Answer from the drawing. Dimensions are ordinates in mm from the lowest x, y and z of the part. Give positions to 0.01 mm unless a question says otherwise; leave off trailing zeros. Order: outer loops, then holes, each group sorted by start corner. A loop starts at its lowest first (then second) coordinate and runs counter-clockwise, first axis right, second up. Notation, with made-up numbers: (25.25, 28) -> (83.25, 28) arc R19 ccw to (83.25, 57) -> close; hole circle Ø7 at (-10.75, 26). An arc over 180 degrees is marked (long way). One line per question, with ' | ' between items. Start each with the question number.
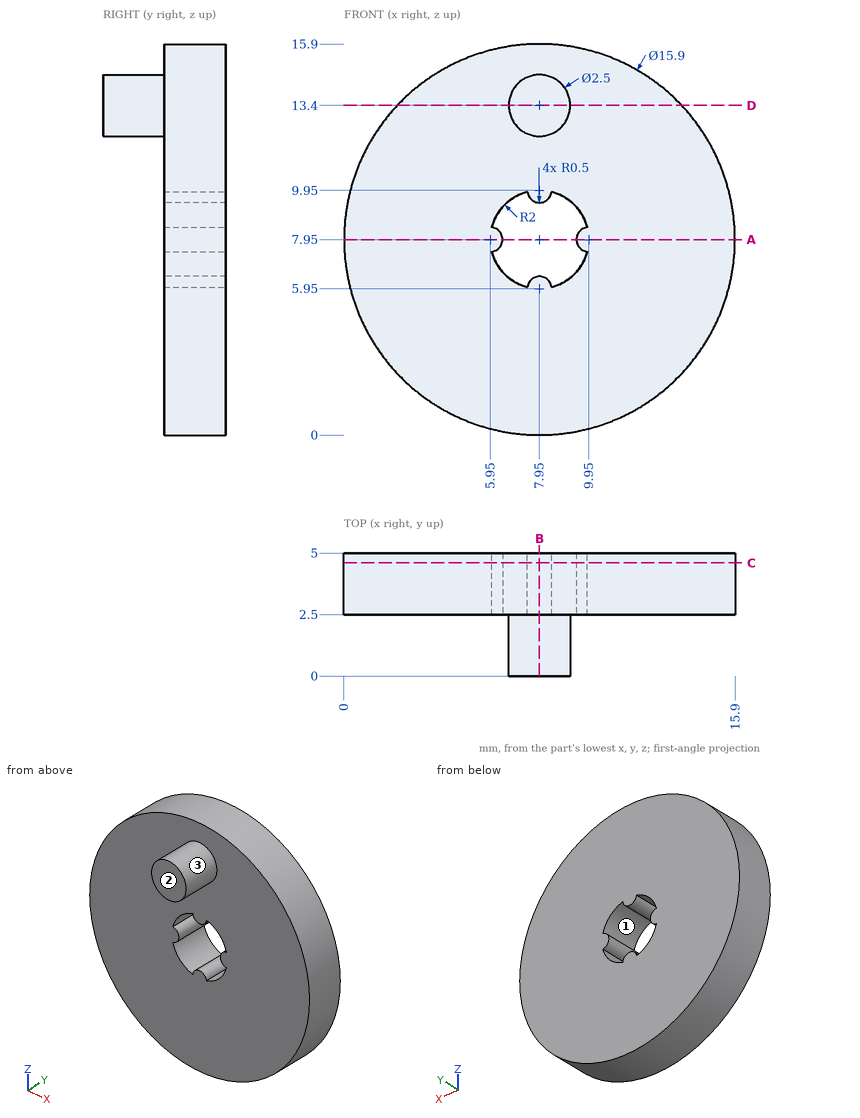
(1) The part is cut by section B-B on x = 7.95. Determine the outline of the cut face in (y, z), plus the area to 3 significant figures.
(2) The part is cut by section A-A on z = 7.95. Determine the outline of the cut face in (x, y).
(3) Given P1, Ø1.5, axis at y = 2, z = 10.5, coming from the -X side; P2, Ø1, axis at x = 10, z = 11, coming from the -Y side, each flat-ended and moving along its own axis, determine where each tip first touches the part or whether it passes through.
(4) The part is cut by section C-C on y = 4.6. Determine the outline of the cut face in (x, z).
(5) The part is cut by section D-D on z = 13.4. Determine the outline of the cut face in (x, y), plus the area to 3 significant figures.
(6) Consider line 1 (Y direction, x = 11.75, z = 3.75); line 2 (Z direction, x = 6.5, y = 4.05); line 3 (X direction, y = 3.25, z = 7). Determine where each line is inside the solid, lowest interval first.
(7) Determine the mould class of the marked faces 1, 2 and 3 for opening direction Z: pulls with the +Z half, pulls with the -Z half, needs draft (parallel to the pull), parting line crosses it, or undercut.
Result sheet:
1) outline: (0, 12.15) -> (2.5, 12.15) -> (2.5, 9.45) -> (5, 9.45) -> (5, 15.9) -> (2.5, 15.9) -> (2.5, 14.65) -> (0, 14.65) -> close; (2.5, 0) -> (5, 0) -> (5, 6.45) -> (2.5, 6.45) -> close | area: 38.5 mm^2
2) outline: (0, 2.5) -> (6.45, 2.5) -> (6.45, 5) -> (0, 5) -> close; (9.45, 2.5) -> (15.9, 2.5) -> (15.9, 5) -> (9.45, 5) -> close
3) P1: stops at x = 0.25 | P2: stops at y = 2.5
4) outline: circle Ø15.9 at (7.95, 7.95); hole (6.01, 7.45) arc R2 ccw to (7.45, 6.01) arc R0.5 cw to (8.45, 6.01) arc R2 ccw to (9.89, 7.45) arc R0.5 cw to (9.89, 8.45) arc R2 ccw to (8.45, 9.89) arc R0.5 cw to (7.45, 9.89) arc R2 ccw to (6.01, 8.45) arc R0.5 cw to start
5) outline: (2.16, 2.5) -> (6.7, 2.5) -> (6.7, 0) -> (9.2, 0) -> (9.2, 2.5) -> (13.74, 2.5) -> (13.74, 5) -> (2.16, 5) -> close | area: 35.2 mm^2
6) line 1: y = 2.5 to 5 | line 2: z = 0.13 to 6.57, 9.33 to 15.77 | line 3: x = 0.06 to 6.19, 9.71 to 15.84
7) face 1: undercut | face 2: needs draft | face 3: parting line crosses it
